Read the model definition and answer for the solid it produces. Units are mm, in the model's axes. Give positions to 0.01 mm unless a question says otherwise; leave off trailing zeros. Loops run counter-clockwise (first coordinate to the right, second up) from the corner with the lowest first, then second, coordinate; pieces in that order, holes last. Notation, with made-up numbers: M -1.5,83.25 L 38.5,83.25 A38 ccw 38.5,121.25 Z; hole C 35.25,52 d2. An arc over 180 degrees is marked long. Return JSON: item names as keys, results as strings. Group by question number.
```python
from build123d import *

# Parameters (mm, degrees)
F0_W     = 50.8
F0_H     = 50.8
F1_DEPTH = 609.6
F2_R     = 15.875
F3_SIZE  = 3.175


with BuildPart() as f1:
    # F0 (on Top) → F1 (new body)
    with BuildSketch(Plane.XY):
        with Locations((25.4, -25.4)):
            Rectangle(F0_W, F0_H)
    extrude(amount=F1_DEPTH)

    # F2
    f2_edges = [f1.edges().sort_by_distance(p)[0] for p in [
        (50.8, 0, 304.8),
    ]]
    fillet(f2_edges, radius=F2_R)

    # F3
    f3_edges = [f1.edges().sort_by_distance(p)[0] for p in [
        (0, 0, 304.8),
        (0, -50.8, 304.8),
        (50.8, -50.8, 304.8),
    ]]
    chamfer(f3_edges, length=F3_SIZE)


solid = f1.part
```
1. Find section A-A (z = 368.5). Write down the section's boundary in (x, y) (3 decimals), and give its area (3 significant figures).
2. Find section B-B (y = -9). Write down the section's boundary in (x, z), and give its area (3 significant figures).
3. Straight lines are drawn through the part: line 1 along X through (y, z) = (-15.5, 153); line 2 along X through (y, z) = (-9.5, 258); line 3 along Y through (x, z) = (37.5, 527). For each, find the intervals that lie inside material, in ascending order.
4. A flat-ended cylindrical pin translates along its axis: P1, Ø10, axis at x = 24.5, y = -16, coming from the -Z side. Find the tip coordinate at first contact, or state that the pin passes through.
Result:
{
 "1": {"outline": "M 0,-47.625 L 3.175,-50.8 L 47.625,-50.8 L 50.8,-47.625 L 50.8,-15.875 A15.875 ccw 34.925,0 L 3.175,0 L 0,-3.175 Z", "area": "2,510 mm2"},
 "2": {"outline": "M 0,0 L 49.23,0 L 49.23,609.6 L 0,609.6 Z", "area": "30,000 mm2"},
 "3": {"line 1": "x = 0 to 50.8", "line 2": "x = 0 to 49.46", "line 3": "y = -50.8 to -0.21"},
 "4": {"P1": "stops at z = 0"}
}
